Can you work these out from the model? Positions are in its coordinate system, mm. A direction names the side the tool comes from. Round coordinates to 2 decimals unless told otherwise and drop trailing zeros. Loops run counter-clockwise (first coordinate to the right, second up) from the corner with the lowest first, then second, coordinate; pieces in that order, holes last. Notation, with made-up numbers: M -32,42.25 L 14,42.25 A23 ccw 14,70.25 Z; hole C 8.25,29 d2. An arc over 180 degrees is marked long. Return JSON: item names as keys, results as strings.
```python
from build123d import *

# Parameters (mm, degrees)
EXTRUDE_1_DEPTH     = 15
SKETCH_2_R          = 6
EXTRUDE_2_DEPTH     = 6
SKETCH_3_R          = 3
CUT_EXTRUDE_1_DEPTH = 28.519640546


with BuildPart() as part:
    # Эскиз1 → Бобышка-Вытянуть1 (new body)
    with BuildSketch(Plane.XY):
        Polygon((10.828570014, 6.721181388), (7.432209439, 10.353476259), (2.90436235, 12.409548224), (-2.065647578, 12.576378965), (-6.721181388, 10.828570014), (-10.353476259, 7.432209439), (-12.409548224, 2.90436235), (-12.576378965, -2.065647578), (-10.828570014, -6.721181388), (-7.432209439, -10.353476259), (-2.90436235, -12.409548224), (2.065647578, -12.576378965), (6.721181388, -10.828570014), (10.353476259, -7.432209439), (12.409548224, -2.90436235), (12.576378965, 2.065647578), align=None)
    extrude(amount=EXTRUDE_1_DEPTH)

    # Эскиз2 → Бобышка-Вытянуть2 (add)
    with BuildSketch(Plane(origin=(0, 0, 0), x_dir=(-1, 0, 0), z_dir=(0, 0, -1))):
        with Locations(Location((0, 0, 0), (0, 0, 180))):
            Circle(SKETCH_2_R)
    extrude(amount=EXTRUDE_2_DEPTH)

    # Эскиз3 → Вырез-Вытянуть1 (cut, through all)
    with BuildSketch(Plane(origin=(0, 0, -6), x_dir=(-1, 0, 0), z_dir=(0, 0, -1))):
        Circle(SKETCH_3_R)
    extrude(amount=-CUT_EXTRUDE_1_DEPTH, mode=Mode.SUBTRACT)


solid = part.part
```
Q1. I'm going to push flat-ended pins straight in: pin 1 Ø8 at (x, z) = (-8.5, -1.5) entering from -Y; pin 2 Ø1.5 at (y, z) = (-7.5, -1.5) entering from -X; pin 3 Ø3 at (y, z) = (9.5, 11) entering from -X; pin 4 Ø4 at (x, z) = (1, -3.5) entering from +Y. Where does each tip first touch, or does it pass through?
Results:
{"pin 1": "stops at y = -11.55", "pin 2": "passes through", "pin 3": "stops at x = -9.75", "pin 4": "stops at y = 6"}
Q2. If I drill on line 1 along Y through (x, z) = (0, -0.25); line 2 along Y through (x, z) = (0, 4.5); line 3 along Z through (x, y) = (2.5, -11), over which ranges is the centre line in solid material (lowest first)?
Results:
{"line 1": "y = -6 to -3, 3 to 6", "line 2": "y = -12.51 to -3, 3 to 12.51", "line 3": "z = 0 to 15"}
Q3. Suppose I cut it at A-A, the plane z = 2.5. Please give me the cut outline in (x, y).
Results:
{"outline": "M -12.58,-2.07 L -10.83,-6.72 L -7.43,-10.35 L -2.9,-12.41 L 2.07,-12.58 L 6.72,-10.83 L 10.35,-7.43 L 12.41,-2.9 L 12.58,2.07 L 10.83,6.72 L 7.43,10.35 L 2.9,12.41 L -2.07,12.58 L -6.72,10.83 L -10.35,7.43 L -12.41,2.9 Z; hole C 0,0 d6"}
Q4. On a 3-axis mill with a long thin cutter (end or side, diameter ignored), from which of +Z, -Z, +X, -X, +Y, -Y can I reach the whole of each face in a straight line? I mean faces 5 (the cylindrical face through (5.723, -1.802, -2.958)), 6 (the flat face through (8.512, -9.154, 7.395)). Say none if no direction works.
Results:
{"face 5": "-Z", "face 6": "+Z, -Z, +X, -Y"}
Q5. Suppose I cut it at B-B, the plane x = 0. Please give me the cut outline in (y, z).
Results:
{"outline": "M -12.51,0 L -6,0 L -6,-6 L -3,-6 L -3,15 L -12.51,15 Z; M 3,-6 L 6,-6 L 6,0 L 12.51,0 L 12.51,15 L 3,15 Z"}
Q6. Suppose I cut it at D-D, the plane x = 4.25. Please give me the cut outline in (y, z), plus the area to 3 significant figures.
Results:
{"outline": "M -11.76,0 L -4.24,0 L -4.24,-6 L 4.24,-6 L 4.24,0 L 11.8,0 L 11.8,15 L -11.76,15 Z", "area": "404 mm2"}
Q7. Thinking about a two-plate mould opening in X: for faces 1 (the flat face through (-9.154, -8.512, 7.395)), 2 (the flat face through (3, -3, 15)), 3 (the cylindrical face through (3, 0, 4)), 4 (the flat face through (11.367, -5.2, 7.395)), which applies, pulls with the +X half, pulls with the -X half, needs draft (parallel to the pull), parting line crosses it, or undercut?
Results:
{"face 1": "pulls with the -X half", "face 2": "needs draft", "face 3": "undercut", "face 4": "pulls with the +X half"}
